```python
from build123d import *

# Parameters (mm, degrees)
GUIDE_BUSH_BARREL_SKETCH_R = 6
GUIDE_BUSH_BARREL_DEPTH    = 10
GUIDE_BUSH_FLANGE_SKETCH_R = 7
GUIDE_BUSH_FLANGE_DEPTH    = 1.05
RUNNING_BORE_SKETCH_R      = 5.05
RUNNING_BORE_DEPTH         = 11.25


with BuildPart() as part:
    # Guide bush barrel sketch → Guide bush barrel (new body)
    with BuildSketch(Plane(origin=(0, -105.98, 0), x_dir=(1, 0, 0), z_dir=(0, 1, 0))):
        with Locations(Location((-20.291651246, 0, 0), (0, 0, 270))):
            Circle(GUIDE_BUSH_BARREL_SKETCH_R)
    extrude(amount=GUIDE_BUSH_BARREL_DEPTH)

    # Guide bush flange sketch → Guide bush flange (add)
    with BuildSketch(Plane(origin=(0, -95.98, 0), x_dir=(1, 0, 0), z_dir=(0, 1, 0))):
        with Locations(Location((-20.291651246, 0, 0), (0, 0, 270))):
            Circle(GUIDE_BUSH_FLANGE_SKETCH_R)
    extrude(amount=GUIDE_BUSH_FLANGE_DEPTH)

    # Running bore sketch → Running bore (cut)
    with BuildSketch(Plane(origin=(0, -106.08, 0), x_dir=(1, 0, 0), z_dir=(0, 1, 0))):
        with Locations(Location((-20.291651246, 0, 0), (0, 0, 90))):
            Circle(RUNNING_BORE_SKETCH_R)
    extrude(amount=RUNNING_BORE_DEPTH, mode=Mode.SUBTRACT)


solid = part.part
```
Check sheet for the modelled part. Datum: model origin and axes. Units: mm. A direction names the side the tool comes from. Round coordinates to 2 decimals unless told otherwise and drop trailing zeros. Loops run counter-clockwise (first coordinate to the right, second up) from the corner with the lowest first, then second, coordinate; pieces in that order, holes last. Notation, with made-up numbers: (55, 88.5) -> (78, 88.5) arc R18 ccw to (78, 101.5) -> close; hole circle Ø2 at (-15, 36). An arc over 180 degrees is marked (long way). Answer in a Markdown table with one row per item.
Q1. Thickness scan on L1, parallel to Z at x = -20.5, y = -103; L2, parallel to Y at x = -23.5, z = -5.75; L3, parallel to X at y = -100.25, z = -4.5. Record the ranges inside material, lowest first.
Data:
| item | result |
|---|---|
| L1 | z = -6 to -5.05, 5.05 to 6 |
| L2 | y = -95.98 to -94.93 |
| L3 | x = -24.26 to -22.58, -18 to -16.32 |
Q2. Sectioned sample at D-D on z = -5.5. Enter the section's corners in (x, y).
Data:
| item | result |
|---|---|
| outline | (-24.62, -95.98) -> (-22.69, -95.98) -> (-22.69, -105.98) -> (-17.89, -105.98) -> (-17.89, -95.98) -> (-15.96, -95.98) -> (-15.96, -94.93) -> (-24.62, -94.93) -> close |
Q3. Release check for a two-part mould opening along X. For faces 3 (the face through (-18, -94.93, 5)), 4 (the face through (-13.35, -95.46, -0.91)), 5 (the face through (-25.3, -100.53, 0.66)) record: released by +X, released by -X, zero draft, split by the parting line, or undercut.
Data:
| item | result |
|---|---|
| face 3 | zero draft |
| face 4 | split by the parting line |
| face 5 | undercut |
Q4. Go/stop test with flat-tipped pins: P1, Ø6, axis at x = -19, y = -104.5, coming from the -Z side; P2, Ø1.5, axis at y = -104, z = 0, coming from the -X side; P3, Ø1.5, axis at x = -17, y = -99, coming from the -Z side. Record where each tip stops, or that it passes through.
Data:
| item | result |
|---|---|
| P1 | stops at z = -6 |
| P2 | stops at x = -26.29 |
| P3 | stops at z = -5.44 |
Q5. Sectioned sample at B-B on x = -18.25. Enter the section's corners in (y, z), then the cut area to 3 significant figures.
Data:
| item | result |
|---|---|
| outline | (-105.98, -5.64) -> (-95.98, -5.64) -> (-95.98, -6.7) -> (-94.93, -6.7) -> (-94.93, -4.62) -> (-105.98, -4.62) -> close; (-105.98, 4.62) -> (-94.93, 4.62) -> (-94.93, 6.7) -> (-95.98, 6.7) -> (-95.98, 5.64) -> (-105.98, 5.64) -> close |
| area | 24.8 mm^2 |
Q6. Sectioned sample at C-C on y = -100.5. Enter the section's corners in (x, z), then the cut area to 3 significant figures.
Data:
| item | result |
|---|---|
| outline | circle Ø12 at (-20.29, 0); hole circle Ø10.1 at (-20.29, 0) |
| area | 33.0 mm^2 |
Q7. Sectioned sample at A-A on z = 0. Enter the section's corners in (x, y), then the cut area to 3 significant figures.
Data:
| item | result |
|---|---|
| outline | (-27.29, -95.98) -> (-26.29, -95.98) -> (-26.29, -105.98) -> (-25.34, -105.98) -> (-25.34, -94.93) -> (-27.29, -94.93) -> close; (-15.24, -105.98) -> (-14.29, -105.98) -> (-14.29, -95.98) -> (-13.29, -95.98) -> (-13.29, -94.93) -> (-15.24, -94.93) -> close |
| area | 23.1 mm^2 |
Q8. Set-up check for faces 1 (the face through (-25, -105.98, -3)), 2 (the face through (-18, -95.98, 6)): record each of +Z, -Z, +X, -X, +Y, -Y from which the full face is reachable in a straight line by a thin tool's end or side.
Data:
| item | result |
|---|---|
| face 1 | +Z, -Z, +X, -X, -Y |
| face 2 | -Y |
